The model under review builds one solid part; all positions refer to its coordinate system, in mm. A direction names the side the tool comes from. Give positions to 0.01 mm unless a question says otherwise; leave off trailing zeros. Loops run counter-clockwise (first coordinate to the right, second up) from the corner with the lowest first, then second, coordinate; pieces in that order, holes last. Notation, with made-up numbers: M 18.5,59 L 62.5,59 A16 cw 62.5,67 Z; hole C -28,15.5 d2. An arc over 180 degrees is marked long. One line per item, written item: value. Start each with the question number.
Q1. To check wall thickness, follow line 1 along Z through (x, y) = (9, -3); line 2 along Y through (x, z) = (0, -0.6); line 3 along Y through (x, z) = (0, -0.3). State the ranges of each line that lie inside material, in increasing order. Write a range as from..to.
Q2. We need section D-D on x = 10. Write out the cut boundary in (y, z).
Q3. We need section A-A on x = 0. Write out the cut boundary in (y, z).
Q4. Mouldability with a two-part tool opening along Z and no side actions: class faces 1 (the face through (11.548, 20.76, 8.419)), 2 (the face through (0.28, 20.748, -0.787)), 3 (the face through (18.5, 20.76, 13.07)), 4 (the face through (14.867, -4.587, -0.74)) as released by +Z, released by -Z, zero draft, split by the parting line, or undercut.
Q5. For faces 5 (the face through (0, 5, 0)), 6 (the face through (-20, 17, -1)), list the 3-axis set-ups (+Z, -Z, +X, -X, +Y, -Y) from which the entire face can be reached by the end or side of a thin tool; tool diameter is ignored.
Q6. For pin 1 (5 mm diameter, centred on x = 10, z = 7, fed in from -Y); pin 2 (3 mm diameter, centred on x = 15.5, y = -4, fed in from +Z); pin 3 (2 mm diameter, centred on y = 18.5, z = 7, fed in from -X), all flat-tipped, find the tip position at first contact; note any pin that passes through.
Q7. We need section B-B on y = -1. Write out the cut boundary in (x, z).
Q8. We need section C-C on z = 8.5. Write out the cut boundary in (x, y), plus the area to 3 significant figures.
```python
from build123d import *

# Parameters (mm, degrees)
SKETCH_1_R                       = 4.25
SM_BASE_FLANGE_1_DEPTH           = 1.5
SM_EDGE_FLANGE_1_STRIP_W         = 8
SM_EDGE_FLANGE_1_STRIP_H         = 1.5
SM_EDGE_FLANGE_1_STRIP_CUT_DEPTH = 40
SM_EDGE_FLANGE_1_DEPTH           = 40
SM_EDGE_FLANGE_1_PROFILE_R       = 2.1
SM_EDGE_FLANGE_1_FLAT_DEPTH      = 1.5


# Sheet-metal steps are written as plain solids
with BuildPart() as part:
    # Sketch 1 → 基体-法兰1 (new body)
    with BuildSketch(Plane.XY):
        with BuildLine():
            Line((-20, 21.5), (20, 21.5))
            Line((20, 21.5), (20, 8))
            ThreePointArc((20, 8), (14.727922061, -4.727922061), (2, -10))
            Line((2, -10), (-2, -10))
            ThreePointArc((-2, -10), (-14.727922061, -4.727922061), (-20, 8))
            Line((-20, 8), (-20, 21.5))
        make_face()
        Circle(SKETCH_1_R, mode=Mode.SUBTRACT)
    extrude(amount=-SM_BASE_FLANGE_1_DEPTH)

    # 边线-法兰1 strip (across the edge) → 边线-法兰1 strip cut (cut)
    with BuildSketch(Plane(origin=(20, 21.5, 0), x_dir=(0, -1, 0), z_dir=(-1, 0, 0))):
        with Locations((-1.5, -0.75)):
            Rectangle(SM_EDGE_FLANGE_1_STRIP_W, SM_EDGE_FLANGE_1_STRIP_H)
    extrude(amount=SM_EDGE_FLANGE_1_STRIP_CUT_DEPTH, mode=Mode.SUBTRACT)

    # 边线-法兰1 bend section (across the edge) → 边线-法兰1 (add)
    with BuildSketch(Plane(origin=(20, 21.5, 0), x_dir=(0, -1, 0), z_dir=(-1, 0, 0))):
        with BuildLine():
            Line((0, 1), (1.5, 1))
            ThreePointArc((1.5, 1), (1.792893219, 0.292893219), (2.5, 0))
            Line((2.5, 0), (2.5, -1.5))
            ThreePointArc((2.5, -1.5), (0.732233047, -0.767766953), (0, 1))
        make_face()
    extrude(amount=SM_EDGE_FLANGE_1_DEPTH)

    # 边线-法兰1 profile (on flange) → 边线-法兰1 flat (add)
    with BuildSketch(Plane(origin=(0, 21.5, 0), x_dir=(-1, 0, 0), z_dir=(0, 1, 0))):
        with BuildLine():
            Line((15, 14.5), (-15, 14.5))
            ThreePointArc((-15, 14.5), (-18.535533906, 13.035533906), (-20, 9.5))
            Line((-20, 9.5), (-20, 1))
            Line((-20, 1), (20, 1))
            Line((20, 1), (20, 9.5))
            ThreePointArc((20, 9.5), (18.535533906, 13.035533906), (15, 14.5))
        make_face()
        with Locations((-10, 7)):
            Circle(SM_EDGE_FLANGE_1_PROFILE_R, mode=Mode.SUBTRACT)
        with Locations((10, 7)):
            Circle(SM_EDGE_FLANGE_1_PROFILE_R, mode=Mode.SUBTRACT)
    extrude(amount=-SM_EDGE_FLANGE_1_FLAT_DEPTH)


solid = part.part
```
Solved:
1. line 1: -1.5..0
1. line 2: -10..-4.25, 4.25..20.92
1. line 3: -10..-4.25, 4.25..21.14
2. outline: M -8.12,-1.5 L 19,-1.5 A2.5 ccw 21.5,1 L 21.5,4.9 L 20,4.9 L 20,1 A1 cw 19,0 L -8.12,0 Z; M 20,9.1 L 21.5,9.1 L 21.5,14.5 L 20,14.5 Z
3. outline: M -10,-1.5 L -4.25,-1.5 L -4.25,0 L -10,0 Z; M 4.25,-1.5 L 19,-1.5 A2.5 ccw 21.5,1 L 21.5,14.5 L 20,14.5 L 20,1 A1 cw 19,0 L 4.25,0 Z
4. face 1: undercut
4. face 2: released by -Z
4. face 3: released by +Z
4. face 4: zero draft
5. face 5: +Z, +X, -X, -Y
5. face 6: +Z, -Z, -X, +Y, -Y
6. pin 1: y = 20
6. pin 2: z = 0
6. pin 3: through
7. outline: M -17.59,-1.5 L -4.13,-1.5 L -4.13,0 L -17.59,0 Z; M 4.13,-1.5 L 17.59,-1.5 L 17.59,0 L 4.13,0 Z
8. outline: M -20,20 L -11.47,20 L -11.47,21.5 L -20,21.5 Z; M -8.53,20 L 8.53,20 L 8.53,21.5 L -8.53,21.5 Z; M 11.47,20 L 20,20 L 20,21.5 L 11.47,21.5 Z
8. area: 51.2 mm2
